```python
from build123d import *

# Parameters (mm, degrees)
SKETCH1_R           = 1.75
SKETCH1_R_2         = 3
BOSS_EXTRUDE3_DEPTH = 4
SKETCH7_R           = 1.3
CUT_EXTRUDE1_DEPTH  = 5


with BuildPart() as part:
    # Sketch1 → Boss-Extrude3 (new body)
    with BuildSketch(Plane.XY):
        with BuildLine():
            ThreePointArc((30.75, -4), (34.75, 0), (30.75, 4))
            Line((30.75, 4), (14.072558403, 4))
            ThreePointArc((14.072558403, 4), (14.06038767, 4.04257326), (14.048088143, 4.085109489))
            ThreePointArc((14.048088143, 4.085109489), (12.709169027, 4.272836063), (11.365584201, 4.122086336))
            ThreePointArc((11.365584201, 4.122086336), (11.169703548, 4.626642697), (10.951436862, 5.12192646))
            ThreePointArc((10.951436862, 5.12192646), (12.008090957, 5.965388247), (12.82210701, 7.044889767))
            ThreePointArc((12.82210701, 7.044889767), (12.669951657, 7.315), (12.51210701, 7.581825517))
            ThreePointArc((12.51210701, 7.581825517), (11.170223244, 7.416617696), (9.911436862, 6.9232593))
            ThreePointArc((9.911436862, 6.9232593), (9.591641884, 7.359925677), (9.252623584, 7.781841479))
            ThreePointArc((9.252623584, 7.781841479), (10.05496909, 8.870045207), (10.561852666, 10.123446462))
            ThreePointArc((10.561852666, 10.123446462), (10.344972209, 10.344972209), (10.123446462, 10.561852666))
            ThreePointArc((10.123446462, 10.561852666), (8.870045207, 10.05496909), (7.781841479, 9.252623584))
            ThreePointArc((7.781841479, 9.252623584), (7.359925677, 9.591641884), (6.9232593, 9.911436862))
            ThreePointArc((6.9232593, 9.911436862), (7.416617696, 11.170223244), (7.581825517, 12.51210701))
            ThreePointArc((7.581825517, 12.51210701), (7.315, 12.669951657), (7.044889767, 12.82210701))
            ThreePointArc((7.044889767, 12.82210701), (5.965388247, 12.008090957), (5.12192646, 10.951436862))
            ThreePointArc((5.12192646, 10.951436862), (4.626642697, 11.169703548), (4.122086336, 11.365584201))
            ThreePointArc((4.122086336, 11.365584201), (4.272836063, 12.709169027), (4.085109489, 14.048088143))
            ThreePointArc((4.085109489, 14.048088143), (3.78652263, 14.131494839), (3.486235477, 14.208555951))
            ThreePointArc((3.486235477, 14.208555951), (2.654199937, 13.14288127), (2.112960617, 11.903927815))
            ThreePointArc((2.112960617, 11.903927815), (1.578061664, 11.986568374), (1.04, 12.04518576))
            ThreePointArc((1.04, 12.04518576), (0.837867713, 13.382005944), (0.31, 14.626715284))
            ThreePointArc((0.31, 14.626715284), (0, 14.63), (-0.31, 14.626715284))
            ThreePointArc((-0.31, 14.626715284), (-0.837867713, 13.382005944), (-1.04, 12.04518576))
            ThreePointArc((-1.04, 12.04518576), (-1.578061664, 11.986568374), (-2.112960617, 11.903927815))
            ThreePointArc((-2.112960617, 11.903927815), (-2.654199937, 13.14288127), (-3.486235477, 14.208555951))
            ThreePointArc((-3.486235477, 14.208555951), (-3.78652263, 14.131494839), (-4.085109489, 14.048088143))
            ThreePointArc((-4.085109489, 14.048088143), (-4.272836063, 12.709169027), (-4.122086336, 11.365584201))
            ThreePointArc((-4.122086336, 11.365584201), (-4.626642697, 11.169703548), (-5.12192646, 10.951436862))
            ThreePointArc((-5.12192646, 10.951436862), (-5.965388247, 12.008090957), (-7.044889767, 12.82210701))
            ThreePointArc((-7.044889767, 12.82210701), (-7.315, 12.669951657), (-7.581825517, 12.51210701))
            ThreePointArc((-7.581825517, 12.51210701), (-7.416617696, 11.170223244), (-6.9232593, 9.911436862))
            ThreePointArc((-6.9232593, 9.911436862), (-7.359925677, 9.591641884), (-7.781841479, 9.252623584))
            ThreePointArc((-7.781841479, 9.252623584), (-8.870045207, 10.05496909), (-10.123446462, 10.561852666))
            ThreePointArc((-10.123446462, 10.561852666), (-10.344972209, 10.344972209), (-10.561852666, 10.123446462))
            ThreePointArc((-10.561852666, 10.123446462), (-10.05496909, 8.870045207), (-9.252623584, 7.781841479))
            ThreePointArc((-9.252623584, 7.781841479), (-9.591641884, 7.359925677), (-9.911436862, 6.9232593))
            ThreePointArc((-9.911436862, 6.9232593), (-11.170223244, 7.416617696), (-12.51210701, 7.581825517))
            ThreePointArc((-12.51210701, 7.581825517), (-12.669951657, 7.315), (-12.82210701, 7.044889767))
            ThreePointArc((-12.82210701, 7.044889767), (-12.008090957, 5.965388247), (-10.951436862, 5.12192646))
            ThreePointArc((-10.951436862, 5.12192646), (-11.169703548, 4.626642697), (-11.365584201, 4.122086336))
            ThreePointArc((-11.365584201, 4.122086336), (-12.709169027, 4.272836063), (-14.048088143, 4.085109489))
            ThreePointArc((-14.048088143, 4.085109489), (-14.131494839, 3.78652263), (-14.208555951, 3.486235477))
            ThreePointArc((-14.208555951, 3.486235477), (-13.14288127, 2.654199937), (-11.903927815, 2.112960617))
            ThreePointArc((-11.903927815, 2.112960617), (-11.986568374, 1.578061664), (-12.04518576, 1.04))
            ThreePointArc((-12.04518576, 1.04), (-13.382005944, 0.837867713), (-14.626715284, 0.31))
            ThreePointArc((-14.626715284, 0.31), (-14.63, 0), (-14.626715284, -0.31))
            ThreePointArc((-14.626715284, -0.31), (-13.382005944, -0.837867713), (-12.04518576, -1.04))
            ThreePointArc((-12.04518576, -1.04), (-11.986568374, -1.578061664), (-11.903927815, -2.112960617))
            ThreePointArc((-11.903927815, -2.112960617), (-13.14288127, -2.654199937), (-14.208555951, -3.486235477))
            ThreePointArc((-14.208555951, -3.486235477), (-14.131494839, -3.78652263), (-14.048088143, -4.085109489))
            ThreePointArc((-14.048088143, -4.085109489), (-12.709169027, -4.272836063), (-11.365584201, -4.122086336))
            ThreePointArc((-11.365584201, -4.122086336), (-11.169703548, -4.626642697), (-10.951436862, -5.12192646))
            ThreePointArc((-10.951436862, -5.12192646), (-12.008090957, -5.965388247), (-12.82210701, -7.044889767))
            ThreePointArc((-12.82210701, -7.044889767), (-12.669951657, -7.315), (-12.51210701, -7.581825517))
            ThreePointArc((-12.51210701, -7.581825517), (-11.170223244, -7.416617696), (-9.911436862, -6.9232593))
            ThreePointArc((-9.911436862, -6.9232593), (-9.591641884, -7.359925677), (-9.252623584, -7.781841479))
            ThreePointArc((-9.252623584, -7.781841479), (-10.05496909, -8.870045207), (-10.561852666, -10.123446462))
            ThreePointArc((-10.561852666, -10.123446462), (-10.344972209, -10.344972209), (-10.123446462, -10.561852666))
            ThreePointArc((-10.123446462, -10.561852666), (-8.870045207, -10.05496909), (-7.781841479, -9.252623584))
            ThreePointArc((-7.781841479, -9.252623584), (3.191677838, -11.661101688), (11.409123542, -4))
            Line((11.409123542, -4), (30.75, -4))
        make_face()
        with Locations((30.75, 0)):
            Circle(SKETCH1_R, mode=Mode.SUBTRACT)
        Circle(SKETCH1_R_2, mode=Mode.SUBTRACT)
    extrude(amount=BOSS_EXTRUDE3_DEPTH)

    # Sketch7 → Cut-Extrude1 (cut, through all)
    with BuildSketch(Plane.XY.offset(4)):
        with Locations((5, 0)):
            Circle(SKETCH7_R)
        with Locations((-5, 0)):
            Circle(SKETCH7_R)
    extrude(amount=-CUT_EXTRUDE1_DEPTH, mode=Mode.SUBTRACT)


solid = part.part
```
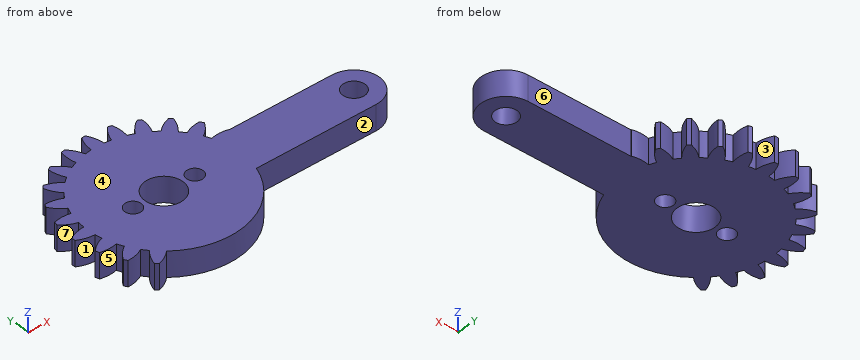
Verification items for the finished model (mm, model axes). Face numbers are marked on the shaded views. A direction names the side the tool comes from. Round coordinates to 2 decimals unless told otherwise and drop trailing zeros. Loops run counter-clockwise (first coordinate to the right, second up) from the corner with the lowest first, then second, coordinate; pieces in that order, holes last. Notation, with made-up numbers: (-8, 64) -> (29, 64) arc R13 ccw to (29, 87) -> close; hole circle Ø11 at (11.25, -1.5). An arc over 180 degrees is marked (long way). Answer as a JSON object with one key per item and string values.
Q1. Section check A-A (z = 0.7). State how many separate pieces and enclosed holes the cut face has, then the cut area to 3 significant figures.
Data:
{"separate pieces": "1", "enclosed holes": "4", "area": "644 mm2"}
Q2. Draft check along Y on the marked faces 1, 2, 3 and 4. Enter one of: pulls with the +Y half, pulls with the -Y half, needs draft (parallel to the pull), parting line crosses it, or undercut.
Data:
{"face 1": "undercut", "face 2": "pulls with the -Y half", "face 3": "pulls with the +Y half", "face 4": "needs draft"}
Q3. Section check B-B (x = 20.5). Record the boundary of the cut face in (y, z).
Data:
{"outline": "(-4, 0) -> (4, 0) -> (4, 4) -> (-4, 4) -> close"}
Q4. Go/stop test with flat-tipped pins: P1, Ø2, axis at x = 21, z = 1.5, coming from the +Y side; P2, Ø2, axis at x = -5, y = 0, coming from the -Z side; P3, Ø1.5, axis at y = 7, z = 3, coming from the +X side; P4, Ø1.5, axis at x = 28.5, z = 1, coming from the -Y side. Record where each tip stops, or that it passes through.
Data:
{"P1": "stops at y = 4", "P2": "passes through", "P3": "stops at x = 12.82", "P4": "stops at y = -4"}
Q5. Access from +Z, -Z, +X, -X, +Y, -Y to the whole of each face (thin tool, end or side, straight path). Record for the marked faces 5, 6 and 7.
Data:
{"face 5": "+Z, -Z", "face 6": "+Z, -Z, +X, +Y", "face 7": "+Z, -Z, -X"}
Q6. Scan lines: line 1 (Y direction, x = 30.75, z = 1.5); line 2 (Y direction, x = 26, z = 1.35); line 3 (X direction, y = -10, z = 3.6). Record each from-to range of solid material in increasing order. Write a range as from..to.
Data:
{"line 1": "y = -4..-1.75, 1.75..4", "line 2": "y = -4..4", "line 3": "x = -10.53..-8.77, -6.79..6.79"}
